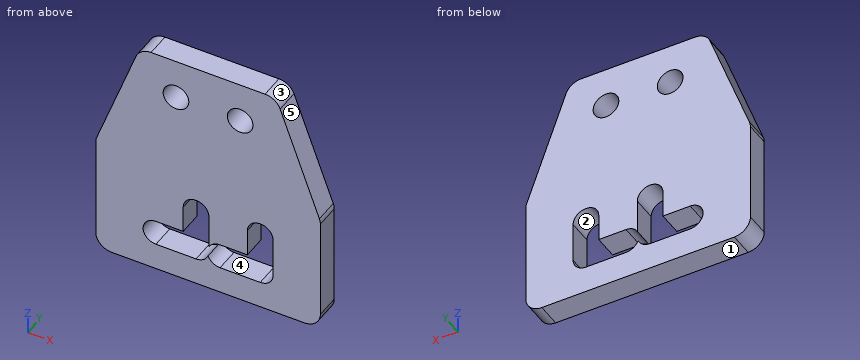
```python
from build123d import *

# Parameters (mm, degrees)
SKETCH1_W           = 28
SKETCH1_H           = 30
BOSS_EXTRUDE1_DEPTH = 3
SKETCH2_R           = 1.6
CUT_EXTRUDE1_DEPTH  = 4
FILLET1_R           = 2


with BuildPart() as part:
    # Sketch1 → Boss-Extrude1 (new body)
    with BuildSketch(Plane(origin=(0, 0, 0), x_dir=(1, 0, 0), z_dir=(0, 1, 0))):
        Rectangle(SKETCH1_W, SKETCH1_H)
        with BuildLine():
            ThreePointArc((1.5, 8.4), (0.687397597, 8.621712173), (0.1, 9.225403331))
            Line((0.1, 9.225403331), (0.1, 5))
            ThreePointArc((0.1, 5), (-1.5, 3.4), (-3.1, 5))
            Line((-3.1, 5), (-3.1, 8.4))
            Line((-3.1, 8.4), (-6.5, 8.4))
            ThreePointArc((-6.5, 8.4), (-8.1, 10), (-6.5, 11.6))
            Line((-6.5, 11.6), (-1.5, 11.6))
            ThreePointArc((-1.5, 11.6), (-0.586447127, 11.313552873), (0, 10.556776436))
            ThreePointArc((0, 10.556776436), (0.586447127, 11.313552873), (1.5, 11.6))
            Line((1.5, 11.6), (6.5, 11.6))
            ThreePointArc((6.5, 11.6), (7.63137085, 11.13137085), (8.1, 10))
            Line((8.1, 10), (8.1, 5))
            ThreePointArc((8.1, 5), (6.5, 3.4), (4.9, 5))
            Line((4.9, 5), (4.9, 8.4))
            Line((4.9, 8.4), (1.5, 8.4))
        make_face(mode=Mode.SUBTRACT)
    extrude(amount=BOSS_EXTRUDE1_DEPTH)

    # Sketch2 → Cut-Extrude1 (cut, through all)
    with BuildSketch(Plane(origin=(0, 3, 0), x_dir=(1, 0, 0), z_dir=(0, 1, 0))):
        with Locations((-4, -10)):
            Circle(SKETCH2_R)
        with Locations((4, -10)):
            Circle(SKETCH2_R)
        Polygon((14, 0), (8.5, -15), (14, -15), align=None)
        Polygon((-8.5, -15), (-14, -15), (-14, 0), align=None)
    extrude(amount=-CUT_EXTRUDE1_DEPTH, mode=Mode.SUBTRACT)

    # Fillet1
    fillet1_edges = [part.edges().sort_by_distance(p)[0] for p in [
        (-14, 1.5, -15),
        (14, 1.5, -15),
        (14, 1.5, 0),
        (8.5, 1.5, 15),
        (-14, 1.5, 0),
        (-8.5, 1.5, 15),
    ]]
    fillet(fillet1_edges, radius=FILLET1_R)


solid = part.part
```
Design review of the part built by this model. Coordinates are the model's own, in mm. Face numbers are marked on the shaded views. A direction names the side the tool comes from. Round coordinates to 2 decimals unless told otherwise and drop trailing zeros. Write each loop counter-clockwise with the first axis right and the second up, starting at its lowest first coordinate (ties: lowest second). Pieces come first, ordered by that corner, then holes.
Item 1: We need section A-A on x = -4. Write out the cut boundary in (y, z).
Item 2: We need section D-D on x = -11.5. Write out the cut boundary in (y, z).
Item 3: We need section C-C on z = 8.75. Write out the cut boundary in (x, y), and give its area (3 significant figures).
Item 4: For the marked faces 4 and 5, list the 3-axis set-ups (+Z, -Z, +X, -X, +Y, -Y) from which the entire face can be reached by the end or side of a thin tool; tool diameter is ignored.
Item 5: For probe 1 along Z at (x, y) = (-4, 1.85); probe 2 along X at (y, z) = (2, -6.25); probe 3 along Z at (x, y) = (-4.5, 1.05), list the stretches that pass through material, from the lowest coordinate up.
Item 6: The part is to be moulded in two halves that separate along X. For the marked faces 1, 2 and 3, say which applies: +X half, -X half, draft (parallel to the pull), parting line (faces both ways), or undercut.
Item 7: We need section B-B on y = 2.4. State how many separate pieces and enclosed holes the cut face has, and give its area (3 significant figures).
Returned:
1. outline: (0, -15) - (3, -15) - (3, -11.6) - (0, -11.6) - close; (0, -8.4) - (3, -8.4) - (3, 8.4) - (0, 8.4) - close; (0, 11.6) - (3, 11.6) - (3, 15) - (0, 15) - close
2. outline: (0, -15) - (3, -15) - (3, 6.82) - (0, 6.82) - close
3. outline: (-10.79, 0) - (-5, 0) - (-5, 3) - (-10.79, 3) - close; (-3, 0) - (3, 0) - (3, 3) - (-3, 3) - close; (5, 0) - (10.79, 0) - (10.79, 3) - (5, 3) - close
3. area: 52.8 mm2
4. face 4: +Y, -Y
4. face 5: +Z, +X, +Y, -Y
5. probe 1: z = -15 to -11.6, -8.4 to 8.4, 11.6 to 15
5. probe 2: x = -14 to -3.1, 0.1 to 4.9, 8.1 to 14
5. probe 3: z = -15 to -11.6, -8.4 to 8.48, 11.52 to 15
6. face 1: draft
6. face 2: undercut
6. face 3: +X half
7. separate pieces: 1
7. enclosed holes: 3
7. area: 660 mm2
